Could you check a few things on this model? Use its own coordinates, in mm. Face numbers are marked on the shaded views. A direction names the side the tool comes from. Give positions to 0.01 mm unless a question says otherwise; leave off trailing zeros. Loops run counter-clockwise (first coordinate to the right, second up) from the corner with the lowest first, then second, coordinate; pieces in that order, holes last. Notation, with made-up numbers: M 83,-20.75 L 118,-20.75 A10 cw 118,-7.75 Z; hole C 67.5,20.25 d2. An arc over 180 degrees is marked long. Use a Markdown table: item, result. Add a question column.
1) Suppose I cut it at B-B on x = 25.5. List the corners of the cut face in (y, z) for me.
2) If I drill on line 1 along Z through (x, y) = (6, 100.5); line 2 along Y through (x, z) = (8.5, -2.5); line 3 along X through (y, z) = (150, 2.5), over which ranges is the centre line in solid material (lowest first)? Write a range as [from, to].
3) Which directions (+Z, -Z, +X, -X, +Y, -Y) give clear straight access to the entire face, cutting with the end or side of a thin tool? Please do the marked faces 1, 2 and 3.
4) Suppose I cut it at A-A on y = 6. List the corners of the cut face in (x, z) for me, and give its area (3 significant figures).
5) Suppose I cut it at C-C on y = 145.5. List the corners of the cut face in (x, z) for me.
6) Will these pins go through, and if not, where does the flat tip stop? pin 1 Ø5 at (x, z) = (-0.5, 4.5) entering from +Y; pin 2 Ø3 at (y, z) = (30.5, -2) entering from +X; pin 3 Ø1 at (y, z) = (140, -4) entering from -X; pin 4 Ø1.5 at (y, z) = (44.5, -3.5) entering from -X.
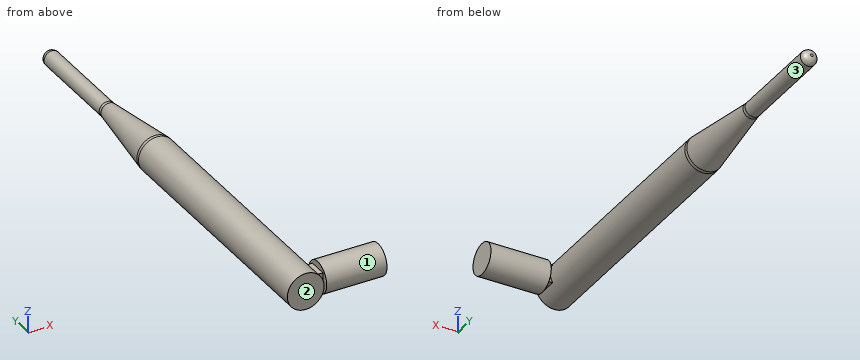
```python
from build123d import *

# Parameters (mm, degrees)
SKETCH3_W           = 23
SKETCH3_H           = 6
SKETCH4_W           = 7
SKETCH4_H           = 7
BOSS_EXTRUDE2_DEPTH = 10


with BuildPart() as part:
    # Sketch2 → Antenna (revolve)
    with BuildSketch(Plane.XY, mode=Mode.PRIVATE) as antenna_sk:
        with BuildLine():
            Line((3, 169.5), (3, 132.622577483))
            ThreePointArc((3, 132.622577483), (3.019323979, 132.001203067), (3.077221233, 131.382230137))
            Line((3.077221233, 131.382230137), (6.922778767, 100.617769863))
            ThreePointArc((6.922778767, 100.617769863), (6.980676021, 99.998796933), (7, 99.377422517))
            Line((7, 99.377422517), (7, 0))
            Line((7, 0), (0, 0))
            Line((0, 0), (0, 172))
            Line((0, 172), (0.5, 172))
            ThreePointArc((0.5, 172), (2.267766953, 171.267766953), (3, 169.5))
        make_face()
    revolve(antenna_sk.sketch.rotate(Axis((0, 0, 0), (0, 1, 0)), 90), axis=Axis((0, 0, 0), (0, 1, 0)))



with BuildPart() as body_2:
    # Sketch3 → Revolve2 (revolve)
    with BuildSketch(Plane.XY, mode=Mode.PRIVATE) as revolve2_sk:
        with Locations((19.5, 3)):
            Rectangle(SKETCH3_W, SKETCH3_H)
    revolve(revolve2_sk.sketch.rotate(Axis((8, 6, 0), (1, 0, 0)), 270), axis=Axis((8, 6, 0), (1, 0, 0)))


with BuildPart() as part_1:
    add(part.part)

    add(body_2.part)  # Boss-Extrude2 merges body 2
    # Sketch4 → Boss-Extrude2 (add)
    with BuildSketch(Plane.ZY.offset(-8)):
        with Locations((0, 6)):
            Rectangle(SKETCH4_W, SKETCH4_H)
    extrude(amount=BOSS_EXTRUDE2_DEPTH)


solid = part_1.part
```
Answer block:
| question | item | result |
|---|---|---|
| 1 | outline | C 6,0 d12 |
| 2 | line 1 | z = [-3.48, 3.48] |
| 2 | line 2 | y = [0.55, 11.45] |
| 2 | line 3 | x = [-1.66, 1.66] |
| 3 | face 1 | +X |
| 3 | face 2 | +Z, -Z, +X, -X, -Y |
| 3 | face 3 | +Y |
| 4 | outline | M 6.06,-3.5 L 8,-3.5 L 8,-6 L 31,-6 L 31,6 L 8,6 L 8,3.5 L 6.06,3.5 A7 ccw long Z |
| 4 | area | 439 mm^2 |
| 5 | outline | C 0,0 d6 |
| 6 | pin 1 | stops at y = 171.48 |
| 6 | pin 2 | stops at x = 6.98 |
| 6 | pin 3 | passes through |
| 6 | pin 4 | stops at x = -6.44 |
